Read the model definition and answer for the solid it produces. Units are mm, in the model's axes. A direction names the side the tool comes from. Give positions to 0.01 mm unless a question says otherwise; leave off trailing zeros. Loops run counter-clockwise (first coordinate to the right, second up) from the corner with the lowest first, then second, coordinate; pieces in that order, holes last. Notation, with made-up numbers: (79, 4.25) - (85, 4.25) arc R33 cw to (85, 42.25) - close; hole circle Ø1 at (-14, 79). An arc over 180 degrees is marked (long way). Put each result on its own line as item: value. Start each with the question number.
1. A cutting plane is placed at D-D, the plane z = 12. Determine the outline of the cut face in (x, y), plus the area to 3 significant figures.
2. A cutting plane is placed at C-C, the plane z = 0. Determine the outline of the cut face in (x, y).
3. For a pull along X with two mould halves and no side action, classify faces 6 (the flat face through (39.5, 10, 0)), 7 (the cylindrical face through (-29.82, 6.03, -13.61)), 8 (the flat face through (-1, 12, 27.5)) as released by +X, released by -X, zero draft, split by the parting line, or undercut.
4. Given pin 1 Ø6 at (x, z) = (-24, 7) entering from -Y; pin 2 Ø14.5 at (x, z) = (-1.5, 1) entering from +Y; pin 3 Ø4.5 at (x, z) = (-19, -14) entering from +Y, each flat-ended and moving along its own axis, determine where each tip first touches the part or whether it passes through.
5. Consider L1, parallel to Z at x = -22, y = 5.5; L2, parallel to X at y = 17.25, z = -4; L3, parallel to Z at x = 12, y = 12.25. Determine where each line is inside the solid, lowest interval first. Write a range as from..to.
6. A cutting plane is placed at B-B, the plane y = 5. Determine the outline of the cut face in (x, z), plus the area to 3 significant figures.
7. A cutting plane is placed at A-A, the plane x = -7.5. Determine the outline of the cut face in (y, z), plus the area to 3 significant figures.
8. For faces 1 (the flat face through (37.98, 21.68, -4.16)), 2 (the flat face through (-6, 6, -15.638)), 3 (the flat face through (-38.021, 20.437, 3.507)), 4 (the flat face through (-5, 1, -9.638)), 5 (the flat face through (-3.922, 22, -18)), determine the directions among +Z, -Z, +X, -X, +Y, -Y from which every point of the face is accessible in a straight line to the end or side of a thin tool.
```python
from build123d import *

# Parameters (mm, degrees)
F0_W      = 79
F0_H      = 55
F0_W_2    = 73
F0_H_2    = 49
F1_DEPTH  = 25
F3_DEPTH  = 79
F0_W_3    = 31
F0_H_3    = 16
F4_DEPTH  = 3
F5_W      = 6
F5_H      = 4
F6_DEPTH  = 3
F5_W_2    = 37
F5_W_3    = 7
F7_DEPTH  = 6
F8_W      = 5
F8_H      = 5
F9_DEPTH  = 12.86194
F10_R     = 1.75
F11_DEPTH = 4


with BuildPart() as f1:
    # F0 (on Front) → F1 (new body)
    with BuildSketch(Plane.XZ):
        Rectangle(F0_W, F0_H)
        Rectangle(F0_W_2, F0_H_2, mode=Mode.SUBTRACT)
    extrude(amount=-F1_DEPTH)

    # F2 (on face) → F3 (cut, through all)
    with BuildSketch(Plane(origin=(-39.5, 0, 0), x_dir=(0, -1, 0), z_dir=(-1, 0, 0))):
        with BuildLine():
            Line((-25, -5), (-18.267742, -3.295049))
            ThreePointArc((-18.267742, -3.295049), (-12.180301, -1.187393), (-16, 4))
            Line((-16, 4), (-16.878049, 3.902439))
            Line((-16.878049, 3.902439), (-25, 3))
            Line((-25, 3), (-25, -5))
        make_face()
    extrude(amount=-F3_DEPTH, mode=Mode.SUBTRACT)

    # F0 (on Front) → F4 (join)
    with BuildSketch(Plane.XZ):
        Rectangle(F0_W_2, F0_H_2)
        with Locations((-4.921641, -1.63806)):
            Rectangle(F0_W_3, F0_H_3, mode=Mode.SUBTRACT)
    extrude(amount=-F4_DEPTH)

    # F5 (on face) → F6 (join)
    with BuildSketch(Plane(origin=(0, 3, 0), x_dir=(-1, 0, 0), z_dir=(0, 1, 0))):
        with Locations((-8.578359, -13.63806)):
            Rectangle(F5_W, F5_H)
    extrude(amount=F6_DEPTH)

    # F5 (on face) → F7 (join)
    with BuildSketch(Plane(origin=(0, 3, 0), x_dir=(-1, 0, 0), z_dir=(0, 1, 0))):
        with Locations((12.921641, -13.63806)):
            Rectangle(F5_W_2, F5_H)
        with Locations((-15.078359, -13.63806)):
            Rectangle(F5_W_3, F5_H)
    extrude(amount=F7_DEPTH)

    # F8 (on face) → F9 (join)
    with BuildSketch(Plane.XY.offset(-24.5)):
        with Locations((-6.421641, 22.5)):
            Rectangle(F8_W, F8_H)
    extrude(amount=F9_DEPTH)

    # F10 (on face) → F11 (cut, through all)
    with BuildSketch(Plane.XY.offset(-11.63806)):
        with Locations((14.828359, 5.95)):
            Circle(F10_R)
        with Locations((-28.071641, 5.95)):
            Circle(F10_R)
    extrude(amount=-F11_DEPTH, mode=Mode.SUBTRACT)


solid = f1.part
```
Return value:
1. outline: (-39.5, 0) - (39.5, 0) - (39.5, 25) - (36.5, 25) - (36.5, 3) - (-36.5, 3) - (-36.5, 25) - (-39.5, 25) - close
1. area: 369 mm2
2. outline: (-39.5, 0) - (-20.42, 0) - (-20.42, 3) - (-36.5, 3) - (-36.5, 12) - (-39.5, 12) - close; (10.58, 0) - (39.5, 0) - (39.5, 12) - (36.5, 12) - (36.5, 3) - (10.58, 3) - close
3. face 6: released by +X
3. face 7: undercut
3. face 8: zero draft
4. pin 1: stops at y = 0
4. pin 2: stops at y = 3
4. pin 3: stops at y = 9
5. L1: z = -27.5..-24.5, -15.64..-11.64, 24.5..27.5
5. L2: x = -39.5..-36.5, 36.5..39.5
5. L3: z = -27.5..-24.5, 24.5..27.5
6. outline: (-39.5, -27.5) - (39.5, -27.5) - (39.5, 27.5) - (-39.5, 27.5) - close; (-31.42, -15.64) - (-29.54, -15.64) - (-29.54, -11.64) - (-31.42, -11.64) - close; (-26.6, -15.64) - (13.36, -15.64) - (13.36, -11.64) - (-26.6, -11.64) - close; (16.3, -15.64) - (18.58, -15.64) - (18.58, -11.64) - (16.3, -11.64) - close; hole (-36.5, -24.5) - (36.5, -24.5) - (36.5, 24.5) - (-36.5, 24.5) - close
6. area: 944 mm2
7. outline: (0, -27.5) - (25, -27.5) - (25, -11.64) - (20, -11.64) - (20, -24.5) - (3, -24.5) - (3, -15.64) - (9, -15.64) - (9, -11.64) - (3, -11.64) - (3, -9.64) - (0, -9.64) - close; (0, 6.36) - (3, 6.36) - (3, 24.5) - (25, 24.5) - (25, 27.5) - (0, 27.5) - close
7. area: 337 mm2
8. face 1: +X, -X, +Y
8. face 2: none
8. face 3: +X, -X
8. face 4: +Y, -Y
8. face 5: +Y
